Could you check a few things on this drawing? It's one solid part, dimensions in mm from its lowest x, y, z. A direction names the side the tool comes from. Round coordinates to 2 decimals unless told otherwise and drop trailing zeros. Order: outer loops, then holes, each group sorted by start corner. A loop starts at its lowest first (then second) coordinate and runs counter-clockwise, first axis right, second up.
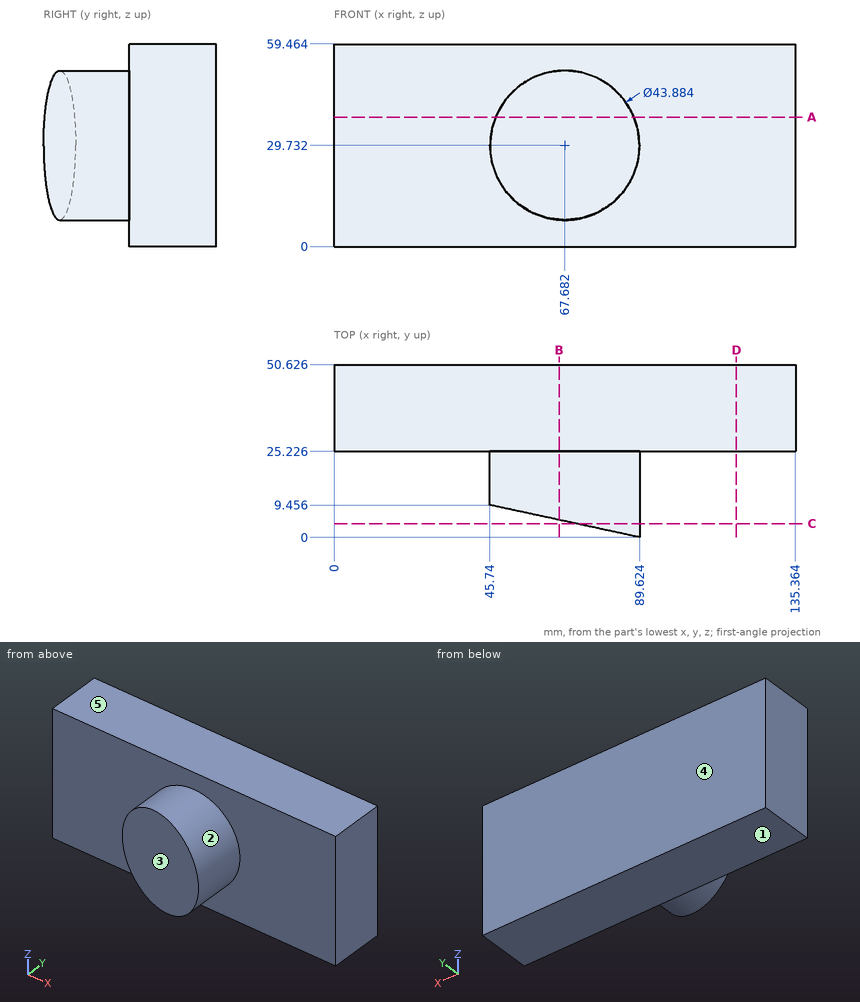
1) If we section it at A-A (z = 38): Write out the boundary of the cut face in (x, y) (1 decimal).
2) For the marked faces 1 and 2, which set-ups out of +Z, -Z, +X, -X, +Y, -Y let a thin tool reach every point of the face, with its end or its side?
3) I need wall thicknesses on line 1 (Y direction, x = 26, z = 34.5); line 2 (X direction, y = 16, z = 22.5) (1 decimal); line 3 (X direction, y = 19.5, z = 24). Which ranges of each line are inside material? Lowest first, please.
4) If we section it at D-D (x = 118): Write out the boundary of the cut face in (y, z).
5) If we section it at C-C (y = 4): Write out the boundary of the cut face in (x, z) (1 decimal), plus the area to 3 significant figures.
6) We'd pull the mould along Y, two halves only. Please class the marked faces 3, 4 and 5: +Y half, -Y half, draft (parallel to the pull), parting line (faces both ways), or undercut.
7) I'm going to push flat-ended pins straight in: pin 1 (10 mm diameter, centred on x = 44, y = 16, fed in from +Z); pin 2 (10 mm diameter, centred on x = 68.5, y = 14, fed in from +Z); pin 3 (8 mm diameter, centred on x = 57, z = 53, fed in from -Y). Where does each tip first touch, or does it pass through?
8) If we section it at B-B (x = 66): Write out the boundary of the cut face in (y, z).
Solutions:
1. outline: (0, 25.2) - (47.4, 25.2) - (47.4, 9.1) - (88, 0.3) - (88, 25.2) - (135.4, 25.2) - (135.4, 50.6) - (0, 50.6) - close
2. face 1: -Z, +X, -X, +Y, -Y
2. face 2: -Y
3. line 1: y = 25.23 to 50.63
3. line 2: x = 47 to 88.4
3. line 3: x = 46.5 to 88.86
4. outline: (25.23, 0) - (50.63, 0) - (50.63, 59.46) - (25.23, 59.46) - close
5. outline: (71.1, 8.1) arc R21.9 ccw to (71.1, 51.4) - close
5. area: 609 mm2
6. face 3: -Y half
6. face 4: +Y half
6. face 5: draft
7. pin 1: stops at z = 41.24
7. pin 2: stops at z = 51.67
7. pin 3: stops at y = 6.4
8. outline: (5.09, 7.85) - (25.23, 7.85) - (25.23, 0) - (50.63, 0) - (50.63, 59.46) - (25.23, 59.46) - (25.23, 51.61) - (5.09, 51.61) - close
